Geometry: final body of the model. Coordinates: model frame, mm. A direction names the side the tool comes from. Give positions to 0.01 mm unless a question says otherwise; leave off trailing zeros. Order: outer loops, then holes, each group sorted by start corner. A loop starts at its lowest first (then second) coordinate and runs counter-clockwise, first axis right, second up. Notation, with made-up numbers: (65.25, -39) -> (116.25, -39) arc R38 ccw to (116.25, 0) -> close; hole circle Ø8 at (32, 9). An arc over 180 degrees is marked (long way). Answer in a Markdown table with one row per item. Add a question column.
Q1. Contact query for flat-ended pins moving along their axis: P1, Ø20.5, axis at x = -30, z = 88, coming from the -Y side; P2, Ø8, axis at x = 59, y = 0, coming from the +Z side; P3, Ø4, axis at y = 1, z = 42.5, coming from the +X side. Output: stop coordinate, or through.
Q2. Cut plane B-B on z = 62. Return the cut outline in (x, y), and give its area (3 significant figures).
Q3. Set-up query: faces 4 (the face through (69.312, 16.752, 12.522)), 5 (the face through (-31.879, 4, 63.686)), 6 (the face through (-19.001, 13, 53)). Return all of +Z, -Z, +X, -X, +Y, -Y with unobstructed straight access to the full face (end or side cutting, diameter ignored); none if empty.
Q4. Cut plane A-A on y = 20. Return the cut outline in (x, z).
Q5. Cut plane D-D on z = 12. Return the cut outline in (x, y).
Q6. Pull-direction query (Y, two-part tool) for faces 1 (the face through (-6, -12.463, 21)), 2 (the face through (9.74, 21.52, 12.52)), 3 (the face through (31, 8, 25.4)); classes: +Y half, -Y half, draft (parallel to the pull), parting line (faces both ways), or undercut.
Q7. Cut plane C-C on x = 63.5. Return the cut outline in (y, z), and give its area (3 significant figures).
Q8. Line query: line 1 along X through (y, z) = (5.5, 23); line 2 along X through (y, z) = (31, 69); line 3 along Y through (x, z) = (61, 5). Output: solid intervals per line, ascending. Write a range as from..to.
from build123d import *

# Parameters (mm, degrees)
F0_R        = 12.7
F1_DEPTH    = 25.4
F2_W        = 25.4
F2_H        = 50.8
F3_DEPTH    = 76.2
F4_R        = 25.4
F5_T1_DEPTH = 152.4
F7_DEPTH    = 25.401
F8_R        = 12.7
F9_R        = 12.69999


# Not quite as in the source:
# - a fillet or chamfer that OpenCascade refuses, or shapes differently, is made with other operations: its cross-section is extruded or revolved along the edge and cut away or added
# - a fillet or chamfer is up to 0.001 mm smaller than in the source, because OpenCascade refuses the exact size


with BuildPart() as f1:
    # F0 (on Top) → F1 (new body)
    with BuildSketch(Plane.XY):
        with BuildLine():
            Line((57.198610294, 38.3368320964), (-44.401389706, 38.3368320964))
            Line((-44.401389706, 38.3368320964), (-44.401389706, -12.4631679036))
            Line((-44.401389706, -12.4631679036), (57.198610294, -12.4631679036))
            ThreePointArc((57.198610294, -12.4631679036), (82.598610294, 12.9368320964), (57.198610294, 38.3368320964))
        make_face()
        with Locations((19.098610294, 12.9368320964)):
            Circle(F0_R, mode=Mode.SUBTRACT)
        with Locations((57.198610294, 12.9368320964)):
            Circle(F0_R, mode=Mode.SUBTRACT)
    extrude(amount=F1_DEPTH)

    # F2 (on face) → F3 (join)
    with BuildSketch(Plane.XY.offset(25.4)):
        with Locations((-31.701389706, 12.9368320964)):
            Rectangle(F2_W, F2_H)
    extrude(amount=F3_DEPTH)

    # F4
    f4_edges = [f1.edges().sort_by_distance(p)[0] for p in [
        (-31.70139, -12.463168, 101.6),
    ]]
    fillet(f4_edges, radius=F4_R)

    # F5: fillet of radius 25.4 on 1 edges, made by hand

    # F5_s2 → F5_t1 (cut)
    with BuildSketch(Plane.YZ.offset(-107.901389706)):
        with BuildLine():
            ThreePointArc((12.9368320964, 101.6), (30.8973443386, 94.1605122421), (38.3368320964, 76.2))
            Line((38.3368320964, 76.2), (38.3368320964, 101.6))
            Line((38.3368320964, 101.6), (12.9368320964, 101.6))
        make_face()
    extrude(amount=F5_T1_DEPTH, mode=Mode.SUBTRACT)

    # F6 (on face) → F7 (cut, through all)
    with BuildSketch(Plane.YZ.offset(-19.001389706)):
        with BuildLine():
            ThreePointArc((12.9368320964, 101.6), (6.3316674028, 100.7261452204), (0.1809873343, 98.1647086118))
            Line((0.1809873343, 98.1647086118), (0.1809873343, 60.0647086118))
            Line((0.1809873343, 60.0647086118), (25.5809873343, 60.0647086118))
            Line((25.5809873343, 60.0647086118), (25.5809873343, 98.2291928659))
            ThreePointArc((25.5809873343, 98.2291928659), (19.4797099497, 100.742834991), (12.9368320964, 101.6))
        make_face()
    extrude(amount=-F7_DEPTH, mode=Mode.SUBTRACT)

    # F8
    f8_edges = [f1.edges().sort_by_distance(p)[0] for p in [
        (-31.70139, 0.180987, 60.064709),
    ]]
    fillet(f8_edges, radius=F8_R)

    # F9 (radius 12.7 in the source; OpenCascade refuses exactly that, so slightly less here)
    f9_edges = [f1.edges().sort_by_distance(p)[0] for p in [
        (-31.70139, 25.580987, 60.064709),
    ]]
    fillet(f9_edges, radius=F9_R)


solid = f1.part
Completed:
| question | item | result |
|---|---|---|
| 1 | P1 | stops at y = -12.42 |
| 1 | P2 | stops at z = 25.4 |
| 1 | P3 | stops at x = -19 |
| 2 | outline | (-44.4, -12.46) -> (-19, -12.46) -> (-19, 6.14) -> (-44.4, 6.14) -> close; (-44.4, 19.62) -> (-19, 19.62) -> (-19, 38.34) -> (-44.4, 38.34) -> close |
| 2 | area | 948 mm² |
| 3 | face 4 | +Z, -Z |
| 3 | face 5 | +Z, +X, -X |
| 3 | face 6 | +Z, +X, +Y, -Y |
| 4 | outline | (-44.4, 0) -> (8.54, 0) -> (8.54, 25.4) -> (-19, 25.4) -> (-19, 62.25) -> (-44.4, 62.25) -> close; (29.65, 0) -> (46.64, 0) -> (46.64, 25.4) -> (29.65, 25.4) -> close; (67.75, 0) -> (81.6, 0) -> (81.6, 25.4) -> (67.75, 25.4) -> close |
| 5 | outline | (-44.4, -12.46) -> (57.2, -12.46) arc R25.4 ccw to (57.2, 38.34) -> (-44.4, 38.34) -> close; hole circle Ø25.4 at (19.1, 12.94); hole circle Ø25.4 at (57.2, 12.94) |
| 6 | face 1 | -Y half |
| 6 | face 2 | undercut |
| 6 | face 3 | draft |
| 7 | outline | (-11.67, 0) -> (1.91, 0) -> (1.91, 25.4) -> (-11.67, 25.4) -> close; (23.96, 0) -> (37.54, 0) -> (37.54, 25.4) -> (23.96, 25.4) -> close |
| 7 | area | 690 mm² |
| 8 | line 1 | x = -44.4..8.8, 29.39..46.9, 67.49..81.49 |
| 8 | line 2 | x = -44.4..-19 |
| 8 | line 3 | y = -12.18..0.82, 25.05..38.05 |
